from build123d import *

# Parameters (mm, degrees)
SKETCH_1_W          = 50
SKETCH_1_H          = 20
SKETCH_1_R          = 1.5
EXTRUDE_1_DEPTH     = 2
FILLET_1_R          = 5
SKETCH_7_W          = 4
SKETCH_7_H          = 17.320508076
CUT_EXTRUDE_1_DEPTH = 8
SKETCH_9_W          = 12
SKETCH_9_H          = 14
EXTRUDE_3_DEPTH     = 1
SKETCH_10_R         = 1.5
CUT_EXTRUDE_2_DEPTH = 1


with BuildPart() as part:
    # 草图1 → 凸台-拉伸1 (new body)
    with BuildSketch(Plane.XY):
        Rectangle(SKETCH_1_W, SKETCH_1_H)
        with Locations((-19.5, 0)):
            Circle(SKETCH_1_R, mode=Mode.SUBTRACT)
        with Locations((19.5, 0)):
            Circle(SKETCH_1_R, mode=Mode.SUBTRACT)
    extrude(amount=EXTRUDE_1_DEPTH)

    # 圆角1
    fillet_1_edges = [part.edges().sort_by_distance(p)[0] for p in [
        (25, -10, 1),
        (-25, -10, 1),
        (-25, 10, 1),
        (25, 10, 1),
    ]]
    fillet(fillet_1_edges, radius=FILLET_1_R)

    # 扫描1: sweep along a path in 草图6
    with BuildLine(Plane(origin=(14, 0, 0), x_dir=(0, 0, -1), z_dir=(1, 0, 0))) as sweep_1_path:
        Line((-2, -4.360392195), (-18.021958635, 4.889889936))
        Line((-18.021958635, 4.889889936), (-25.591084209, 18))
        Line((-25.591084209, 18), (-25.591084209, 22))
    # 草图2 → 扫描1 (sweep)
    with BuildSketch(Plane.XY.offset(2)):
        Polygon((14, 4), (12, -6), (16, -6), align=None)
    sweep_1 = sweep(path=sweep_1_path.line, transition=Transition.RIGHT)

    # 草图7 → 切除-拉伸1 (cut)
    with BuildSketch(Plane(origin=(0, 20, 0), x_dir=(1, 0, 0), z_dir=(0, 1, 0))):
        with Locations((14, -18.350772183)):
            Rectangle(SKETCH_7_W, SKETCH_7_H)
    cut_extrude_1 = extrude(amount=CUT_EXTRUDE_1_DEPTH, mode=Mode.SUBTRACT)

    # 草图9 → 凸台-拉伸3 (add)
    with BuildSketch(Plane(origin=(0, 20, 0), x_dir=(1, 0, 0), z_dir=(0, 1, 0))):
        with Locations((14, -22.429425186)):
            Rectangle(SKETCH_9_W, SKETCH_9_H)
    extrude_3 = extrude(amount=EXTRUDE_3_DEPTH)

    # 草图10 → 切除-拉伸2 (cut)
    with BuildSketch(Plane(origin=(0, 21, 0), x_dir=(1, 0, 0), z_dir=(0, 1, 0))):
        with Locations(Location((11, -25.929425186, 0), (0, 0, 270))):
            Circle(SKETCH_10_R)
        with Locations(Location((17, -18.929425186, 0), (0, 0, 270))):
            Circle(SKETCH_10_R)
        with Locations(Location((11, -18.929425186, 0), (0, 0, 270))):
            Circle(SKETCH_10_R)
        with Locations(Location((17, -25.929425186, 0), (0, 0, 270))):
            Circle(SKETCH_10_R)
    cut_extrude_2 = extrude(amount=-CUT_EXTRUDE_2_DEPTH, mode=Mode.SUBTRACT)

    # 镜向1: 扫描1, 切除-拉伸1, 凸台-拉伸3, 切除-拉伸2 across plane
    add(sweep_1.mirror(Plane(origin=(0, 0, 0), x_dir=(0, 0, 1), z_dir=(1, 0, 0))))
    add(cut_extrude_1.mirror(Plane(origin=(0, 0, 0), x_dir=(0, 0, 1), z_dir=(1, 0, 0))), mode=Mode.SUBTRACT)
    add(extrude_3.mirror(Plane(origin=(0, 0, 0), x_dir=(0, 0, 1), z_dir=(1, 0, 0))))
    add(cut_extrude_2.mirror(Plane(origin=(0, 0, 0), x_dir=(0, 0, 1), z_dir=(1, 0, 0))), mode=Mode.SUBTRACT)


solid = part.part
Model file for the job. Use its own axes, mm. A direction names the side the tool comes from. Give positions to 0.01 mm unless a question says otherwise; leave off trailing zeros. Order: outer loops, then holes, each group sorted by start corner. A loop starts at its lowest first (then second) coordinate and runs counter-clockwise, first axis right, second up. Notation, with made-up numbers: M 21.25,-33 L 61.25,-33 A19 cw 61.25,-14 Z; hole C -27,65 d9. An arc over 180 degrees is marked long. Write item = value, one per line.
Q1. Drill centre lines: line 1 (Z direction, x = -17, y = 20.55); line 2 (Y direction, x = 19.5, z = 1.35); line 3 (Y direction, x = 8.5, z = 25.5). Where is each one in solid material? Low to high. Write a range as [from, to].
Derived:
line_1 = [15.43, 17.43], [20.43, 24.43], [27.43, 29.43]
line_2 = [-10, -1.5], [1.5, 10]
line_3 = [20, 21]
Q2. Cut at A-A, the plane x = -11. List the corners of the cut face in (y, z).
Derived:
outline = M -10,0 L 10,0 L 10,2 L -10,2 Z; M 20,15.43 L 21,15.43 L 21,17.43 L 20,17.43 Z; M 20,20.43 L 21,20.43 L 21,24.43 L 20,24.43 Z; M 20,27.43 L 21,27.43 L 21,29.43 L 20,29.43 Z
Q3. Tool access for faces 4 (the flat face through (-15.057, 11.983, 19.042)), 5 (the flat face through (-8, 20.5, 22.5)), 6 (the flat face through (12.983, 12.155, 18.943)), 7 (the flat face through (-15.31, 19.2, 24.03)): list every direction of +Z, -Z, +X, -X, +Y, -Y with a clear straight run to the whole face (end or side of a thin tool).
Derived:
face_4 = -X
face_5 = +Z, -Z, +Y, -Y
face_6 = none
face_7 = -Z, -X
Q4. Cut at B-B, the plane y = 0. List the corners of the cut face in (x, z), then the cut area to 3 significant figures.
Derived:
outline = M -25,0 L -21,0 L -21,2 L -25,2 Z; M -18,0 L 18,0 L 18,2 L 14.8,2 L 16,12.39 L 12,12.39 L 13.2,2 L -13.2,2 L -12,12.39 L -16,12.39 L -14.8,2 L -18,2 Z; M 21,0 L 25,0 L 25,2 L 21,2 Z
area = 146 mm2
Q5. Cut at C-C, the plane z = 16.5. List the corners of the cut face in (x, y), then the cut area to 3 significant figures.
Derived:
outline = M -20,20 L -8,20 L -8,21 L -20,21 Z; M -16,2.37 L -12,2.37 L -12.81,6.41 L -14,16.73 L -15.19,6.41 Z; M 8,20 L 20,20 L 20,21 L 8,21 Z; M 12,2.37 L 16,2.37 L 15.19,6.41 L 14,16.73 L 12.81,6.41 Z
area = 74.4 mm2
Q6. Cut at D-D, the plane z = 9.5. List the corners of the cut face in (x, y), then the cut area to 3 significant figures.
Derived:
outline = M -16,-1.67 L -12,-1.67 L -14,8.33 Z; M 12,-1.67 L 16,-1.67 L 14,8.33 Z
area = 40.0 mm2
Q7. Two-plate mould, pull along Y, no slides. Class faces 1 (the flat face through (-13, 20, 22)), 2 (the flat face through (0, -10, 1)), 3 (the cylindrical face through (-11.45, 20.51, 20.36)): pulls with the +Y half, pulls with the -Y half, needs draft (parallel to the pull), parting line crosses it, or undercut.
Derived:
face_1 = undercut
face_2 = pulls with the -Y half
face_3 = needs draft
Q8. Flat gauge pins, fed straight in: pin 1 (1.6 mm diameter, centred on x = 9.5, z = 1, fed in from +Y); pin 2 (6 mm diameter, centred on y = 7.5, z = 19.5, fed in from -X); pin 3 (3 mm diameter, centred on x = -10, y = 5.5, fed in from +Z). Where does each tip first touch, or does it go through?
Derived:
pin_1 = 10
pin_2 = -16
pin_3 = 2
